Can you work these out from the model? Positions are in its coordinate system, mm. Face numbers are marked on the shaded views. A direction names the side the tool comes from. Round coordinates to 2 decimals unless told otherwise and drop trailing zeros. Loops run counter-clockwise (first coordinate to the right, second up) from the corner with the lowest first, then second, coordinate; pieces in that order, holes last. Notation, with made-up numbers: M 79.25,84.25 L 101.25,84.25 A22 cw 101.25,106.25 Z; hole C -28,-31.5 d3. An arc over 180 degrees is marked long. Answer as CSV lines item,"result".
from build123d import *

# Parameters (mm, degrees)
F0_R     = 11
F0_R_2   = 8.05
F1_DEPTH = 2
F2_R     = 10.25
F2_R_2   = 8.05
F3_DEPTH = 10
F4_SIZE2 = 0.6994614872
F4_SIZE  = 1.5


with BuildPart() as f1:
    # F0 (on Top) → F1 (new body)
    with BuildSketch(Plane.XY):
        Circle(F0_R)
        Circle(F0_R_2, mode=Mode.SUBTRACT)
    extrude(amount=F1_DEPTH)

    # F2 (on face) → F3 (join)
    with BuildSketch(Plane.XY.offset(2)):
        Circle(F2_R)
        Circle(F2_R_2, mode=Mode.SUBTRACT)
    extrude(amount=F3_DEPTH)

    # F4
    f4_edges = [f1.edges().sort_by_distance(p)[0] for p in [
        (-8.05, 0, 12),
    ]]
    f4_side = f1.faces().sort_by_distance((-8.05, 0, 6))[0]
    chamfer(f4_edges, length=F4_SIZE, length2=F4_SIZE2, reference=f4_side)


solid = f1.part
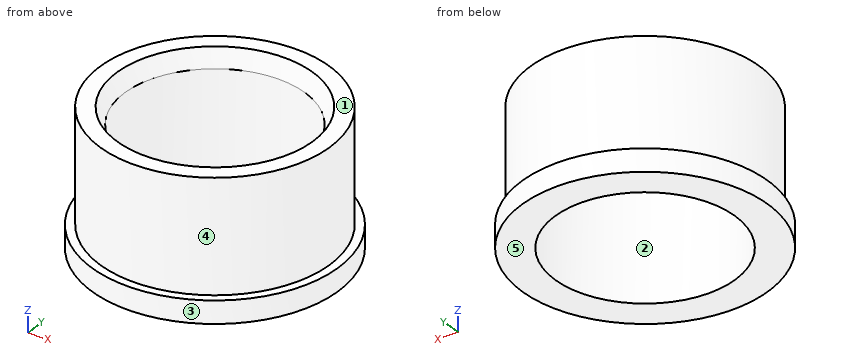
Item 1: If I drill on line 1 along Y through (x, z) = (0, 5); line 2 along Y through (x, z) = (-4.75, 4); line 3 along X through (y, z) = (7.25, 4), over which ranges is the centre line in solid material (lowest first)? Write a range as from..to.
Output:
line 1,"y = -10.25..-8.05, 8.05..10.25"
line 2,"y = -9.08..-6.5, 6.5..9.08"
line 3,"x = -7.25..-3.5, 3.5..7.25"
Item 2: If we section it at C-C on z = 8: Write out the boundary of the cut face in (x, y).
Output:
outline,"C 0,0 d20.5; hole C 0,0 d16.1"
Item 3: Will these pins go through, and if not, where does the flat tip stop? pin 1 (1 mm diameter, centred on x = -1.5, z = 3.5, fed in from -Y); pin 2 (5 mm diameter, centred on x = 5.5, y = 4, fed in from -Z).
Output:
pin 1,"stops at y = -10.2"
pin 2,"stops at z = 0"
Item 4: If we section it at D-D on y = -9.25: Write out the boundary of the cut face in (x, z), then the cut area to 3 significant figures.
Output:
outline,"M -5.95,0 L 5.95,0 L 5.95,2 L 4.42,2 L 4.42,12 L -4.42,12 L -4.42,2 L -5.95,2 Z"
area,"112 mm2"
Item 5: We'd pull the mould along X, two halves only. Please class the marked faces 1, 2 and 3: released by +X, released by -X, zero draft, split by the parting line, or undercut.
Output:
face 1,"zero draft"
face 2,"undercut"
face 3,"split by the parting line"
Item 6: If we section it at A-A on y = 0: Write out the boundary of the cut face in (x, z), then the cut area to 3 significant figures.
Output:
outline,"M -11,0 L -8.05,0 L -8.05,10.5 L -8.75,12 L -10.25,12 L -10.25,2 L -11,2 Z; M 8.05,0 L 11,0 L 11,2 L 10.25,2 L 10.25,12 L 8.75,12 L 8.05,10.5 Z"
area,"54.8 mm2"
Item 7: On a 3-axis mill with a long thin cutter (end or side, diameter ignored), from which of +Z, -Z, +X, -X, +Y, -Y can I reach the whole of each face in a straight line? I mean the marked faces 4 and 5. Say none if no direction works.
Output:
face 4,"+Z"
face 5,"-Z, +X, -X, +Y, -Y"
